For this review, take the finished solid that the model builds, in its own axes (mm). A direction names the side the tool comes from. Give positions to 0.01 mm unless a question says otherwise; leave off trailing zeros. Order: outer loops, then holes, each group sorted by start corner. A loop starts at its lowest first (then second) coordinate and runs counter-clockwise, first axis right, second up.
from build123d import *

# Parameters (mm, degrees)
F1_DEPTH  = 5.08
F3_DEPTH  = 2.286
F5_DEPTH  = 17.78
F6_SIZE   = 5.08
F7_R      = 1.4
F8_DEPTH  = 12.7
F10_DEPTH = 5.08


with BuildPart() as f1:
    # F0 (on Top) → F1 (new body)
    with BuildSketch(Plane.XY):
        Polygon((-17.894535, 19.113216), (-17.894535, 2.39155), (-17.894535, -10.837617), (13.855465, -10.837617), (13.855465, 10.752383), (13.855465, 32.342383), (-17.894535, 32.342383), align=None)
    extrude(amount=F1_DEPTH)

    # F2 (on face) → F3 (join)
    with BuildSketch(Plane.XY.offset(5.08)):
        with BuildLine():
            Line((-2.554535, 20.812383), (-17.894535, 20.812383))
            Line((-17.894535, 20.812383), (-17.894535, 0.692383))
            Line((-17.894535, 0.692383), (-2.554535, 0.692383))
            ThreePointArc((-2.554535, 0.692383), (7.505465, 10.752383), (-2.554535, 20.812383))
        make_face()
    extrude(amount=F3_DEPTH)

    # F4 (on face) → F5 (join)
    with BuildSketch(Plane.XY.offset(7.366)):
        with BuildLine():
            Line((-2.554535, 20.812383), (-17.894535, 20.812383))
            Line((-17.894535, 20.812383), (-17.894535, 0.692383))
            Line((-17.894535, 0.692383), (-2.554535, 0.692383))
            ThreePointArc((-2.554535, 0.692383), (7.505465, 10.752383), (-2.554535, 20.812383))
        make_face()
        with BuildLine():
            Line((13.855465, 32.342383), (-17.894535, 32.342383))
            Line((-17.894535, 32.342383), (-17.894535, 20.812383))
            Line((-17.894535, 20.812383), (-2.554535, 20.812383))
            ThreePointArc((-2.554535, 20.812383), (7.505465, 10.752383), (-2.554535, 0.692383))
            Line((-2.554535, 0.692383), (-17.894535, 0.692383))
            Line((-17.894535, 0.692383), (-17.894535, -10.837617))
            Line((-17.894535, -10.837617), (13.855465, -10.837617))
            Line((13.855465, -10.837617), (13.855465, 32.342383))
        make_face()
    extrude(amount=F5_DEPTH)

    # F6
    f6_edges = [f1.edges().sort_by_distance(p)[0] for p in [
        (13.855465, -10.837617, 16.256),
        (13.855465, -10.837617, 2.54),
        (13.855465, 32.342383, 16.256),
        (13.855465, 32.342383, 2.54),
    ]]
    chamfer(f6_edges, length=F6_SIZE)

    # F7 (on face) → F8 (cut)
    with BuildSketch(Plane.XY.offset(25.146)):
        with BuildLine():
            Line((-4.438033, 25.391014), (-17.894535, 25.391014))
            Line((-17.894535, 25.391014), (-17.894535, -3.048986))
            Line((-17.894535, -3.048986), (-4.438033, -3.048986))
            ThreePointArc((-4.438033, -3.048986), (9.781967, 11.171014), (-4.438033, 25.391014))
        make_face()
        with Locations((-11.544535, 28.532383)):
            Circle(F7_R)
        with Locations((4.965465, 28.532383)):
            Circle(F7_R)
        with Locations((-11.544535, -7.027617)):
            Circle(F7_R)
        with Locations((4.965465, -7.027617)):
            Circle(F7_R)
    extrude(amount=-F8_DEPTH, mode=Mode.SUBTRACT)

    # F9 (on face) → F10 (cut)
    with BuildSketch(Plane.XY.offset(12.446)):
        with BuildLine():
            Line((-4.438033, 26.661014), (-19.164535, 26.661014))
            Line((-19.164535, 26.661014), (-19.164535, -4.318986))
            Line((-19.164535, -4.318986), (-4.438033, -4.318986))
            ThreePointArc((-4.438033, -4.318986), (11.051967, 11.171014), (-4.438033, 26.661014))
        make_face()
    extrude(amount=F10_DEPTH, mode=Mode.SUBTRACT)


solid = f1.part
1) Clearance check with flat-ended pins moving along their axes: pin 1 (2 mm diameter, centred on x = -11.54, y = -7.03, fed in from +Z); pin 2 (2 mm diameter, centred on x = 4.97, y = -7.03, fed in from -Z); pin 3 (0.7 mm diameter, centred on x = -7, z = 6, fed in from +Y). State where each tip first meets the part, or that it passes through.
Answer sheet:
pin 1: stops at z = 12.45
pin 2: stops at z = 0
pin 3: stops at y = 20.81
2) Tool access review of faces 1 (the face through (-10, 0.692, 6)), 2 (the face through (-2, 11, 0)), 3 (the face through (-11, -4.319, 15)), 4 (the face through (5, -7, 12.446)): name each direction out of +Z, -Z, +X, -X, +Y, -Y from which nothing blocks a thin tool from reaching the whole face with its end or side.
Answer sheet:
face 1: +X, -X, -Y
face 2: -Z, +X, -X, +Y, -Y
face 3: -X
face 4: +Z
3) We need section A-A on y = -2.5. Give the boundary of the cut face in (x, z) (3 decimals), then the cut area to 3 significant figures.
Answer sheet:
outline: (-17.895, 0) - (13.855, 0) - (13.855, 5.08) - (-17.895, 5.08) - close; (-17.895, 7.366) - (13.855, 7.366) - (13.855, 25.146) - (-0.525, 25.146) - (-0.525, 17.526) - (2.845, 17.526) - (2.845, 12.446) - (-17.895, 12.446) - close
area: 488 mm2
4) We need section C-C on z = 19.75. Give the boundary of the cut face in (x, y), then the cut area to 3 significant figures.
Answer sheet:
outline: (-17.89, -10.84) - (8.78, -10.84) - (13.86, -5.76) - (13.86, 27.26) - (8.78, 32.34) - (-17.89, 32.34) - (-17.89, 25.39) - (-4.44, 25.39) arc R14.22 cw to (-4.44, -3.05) - (-17.89, -3.05) - close; hole circle Ø2.8 at (-11.54, -7.03); hole circle Ø2.8 at (-11.54, 28.53); hole circle Ø2.8 at (4.97, -7.03); hole circle Ø2.8 at (4.97, 28.53)
area: 620 mm2
5) To check wall thickness, follow line 1 (Y direction, x = -7.5, z = 19.25); line 2 (Y direction, x = -7, z = 13); line 3 (Y direction, x = 4, z = 20). State the ranges of each line that lie inside material, in increasing order.
Answer sheet:
line 1: y = -10.84 to -3.05, 25.39 to 32.34
line 2: y = -10.84 to -4.32, 26.66 to 32.34
line 3: y = -10.84 to -8.04, -6.01 to -0.27, 22.62 to 27.52, 29.55 to 32.34
6) We need section D-D on z = 10.25. Give the boundary of the cut face in (x, y).
Answer sheet:
outline: (-17.89, -10.84) - (8.78, -10.84) - (13.86, -5.76) - (13.86, 27.26) - (8.78, 32.34) - (-17.89, 32.34) - close
7) Draft analysis for pull direction Y (two halves, no side actions). For faces 5 (the face through (11.05, 10.83, 14.95)), 6 (the face through (-10, 20.812, 6)), 7 (the face through (12, 11, 25.146)), 8 (the face through (-11, -3.049, 21)), state which applies: +Y half, -Y half, draft (parallel to the pull), parting line (faces both ways), or undercut.
Answer sheet:
face 5: undercut
face 6: +Y half
face 7: draft
face 8: undercut
8) We need section B-B on x = -15.5. Give the boundary of the cut face in (y, z).
Answer sheet:
outline: (-10.84, 0) - (32.34, 0) - (32.34, 5.08) - (20.81, 5.08) - (20.81, 7.37) - (32.34, 7.37) - (32.34, 25.15) - (25.39, 25.15) - (25.39, 17.53) - (26.66, 17.53) - (26.66, 12.45) - (-4.32, 12.45) - (-4.32, 17.53) - (-3.05, 17.53) - (-3.05, 25.15) - (-10.84, 25.15) - (-10.84, 7.37) - (0.69, 7.37) - (0.69, 5.08) - (-10.84, 5.08) - close
